Build history of the part. All positions in model axes, mm. A direction names the side the tool comes from. Round coordinates to 2 decimals unless told otherwise and drop trailing zeros. Write each loop counter-clockwise with the first axis right and the second up, starting at its lowest first coordinate (ties: lowest second). Pieces come first, ordered by that corner, then holes. Notation, with made-up numbers: M 40,14.25 L 62,14.25 A25 cw 62,44.25 Z; hole C 55.5,76.5 d4. An arc over 180 degrees is marked long. Write item = value, one per line.
Autodesk Fusion 360 part; units mm, degrees
sketch "Sketch1" plane through (0, 0, 0) normal (0, 1, 0) x (1, 0, 0)
  line L0 (-12.25, 0) -> (0, 0)
  line L1 (0, 0) -> (0, -15.7252) construction
  arc A0 (-12.25, 0) -> (-7, -11) centre (0, -0.9062) ccw
  arc A1 (-8.2142, -6.2319) -> (-7, -11) centre (26.2265, 0) ccw
  arc A2 (-3.925, -3.5) -> (-6.6248, -3.9119) centre (0, -38.2792) ccw
  line L2 (-3.925, -3.5) -> (-3.75, -5.5)
  line L3 (-3.75, -5.5) -> (-0.75, -5.5)
  arc A3 (-6.6248, -3.9119) -> (-8.2142, -6.2319) centre (-6.2462, -5.8758) ccw
  line L4 (-2.25, -5.5) -> (-2.25, 0) construction
  line L5 (-0.575, -3.5) -> (-0.75, -5.5)
  arc A4 (0, -3.4953) -> (-0.575, -3.5) centre (0, -38.4953) ccw
  arc A5 (8.2142, -6.2319) -> (6.6248, -3.9119) centre (6.2462, -5.8758) ccw
  arc A6 (7, -11) -> (8.2142, -6.2319) centre (-26.2265, 0) ccw
  arc A7 (7, -11) -> (12.25, 0) centre (0, -0.9062) ccw
  line L6 (12.25, 0) -> (0, 0)
  arc A8 (6.6248, -3.9119) -> (3.925, -3.5) centre (0, -38.2792) ccw
  line L7 (3.925, -3.5) -> (3.75, -5.5)
  line L8 (3.75, -5.5) -> (0.75, -5.5)
  line L9 (0.575, -3.5) -> (0.75, -5.5)
  arc A9 (0.575, -3.5) -> (0, -3.4953) centre (0, -38.4953) ccw
  dimension "d1" = 12.25
  dimension "d3" = 11
  dimension "d4" = 7
  dimension "d6" = 2
  dimension "d7" = 95
  dimension "d8" = 3
  dimension "d9" = 0.75
  dimension "d10" = 35
  dimension "d11" = 5.5
  dimension "d12" = 2
extrude "Extrude1" add sketch "Sketch1" along normal blind 150
equation "d1 = ( 24.5 / 2 ) * 1 mm"
equation "d4 = ( 14 / 2 ) * 1 mm"
equation "d7 = 90 deg + 5 deg"
equation "d9 = ( 1.5 / 2 ) * 1 mm"
1. Tool access for faces 4 (the face through (0, 74, 0)), 5 (the face through (-5.298, 73.95, 3.682)), 6 (the face through (-7.682, 73.95, 8.671)): list every direction of +Z, -Z, +X, -X, +Y, -Y with a clear straight run to the whole face (end or side of a thin tool).
Responses:
face_4 = -Z, +X, -X, +Y, -Y
face_5 = +Z, +Y, -Y
face_6 = +Y, -Y
2. Mould opens along Z. For faces 1 (the face through (5.26, 73.95, 3.677)), 2 (the face through (0, 0, 3)), 3 (the face through (7.884, 73.95, 4.727)) say: pulls with the +Z half, pulls with the -Z half, needs draft (parallel to the pull), parting line crosses it, or undercut.
Responses:
face_1 = pulls with the +Z half
face_2 = needs draft
face_3 = undercut
3. Probe probe 1 along X at (y, z) = (33, 4.75); probe 2 along Z at (x, y) = (3.5, 72.5); probe 3 along X at (y, z) = (105, 8.75). List the from-to ranges inside material, lowest first.
Responses:
probe_1 = -11.67 to -7.9, -3.82 to -0.68, 0.68 to 3.82, 7.9 to 11.67
probe_2 = 0 to 5.5
probe_3 = -9.45 to -7.66, 7.66 to 9.45
4. Band-saw the part on C-C (x = -2). List the corners of the cut face in (y, z).
Responses:
outline = M 0,0 L 150,0 L 150,5.5 L 0,5.5 Z
5. Band-saw the part on D-D (x = -10.5). List the corners of the cut face in (y, z).
Responses:
outline = M 0,0 L 150,0 L 150,7.28 L 0,7.28 Z
6. Band-saw the part on A-A (z = 9.5). List the corners of the cut face in (x, y), plus the area to 3 significant figures.
Responses:
outline = M -8.78,0 L -7.46,0 L -7.46,150 L -8.78,150 Z; M 7.46,0 L 8.78,0 L 8.78,150 L 7.46,150 Z
area = 395 mm²
7. Flat gauge pins, fed straight in: pin 1 (1 mm diameter, centred on y = 115, z = 9, fed in from -X) (3 decimals); pin 2 (4 mm diameter, centred on x = 2, y = 81.5, fed in from +Z); pin 3 (3 mm diameter, centred on x = 9.5, y = 80.5, fed in from -Z); pin 4 (1.5 mm diameter, centred on y = 55.5, z = 7, fed in from +X). Where does each tip first touch, or does it go through?
Responses:
pin_1 = -9.655
pin_2 = 5.5
pin_3 = 0
pin_4 = 11.06
